For this review, take the finished solid that the model builds, in its own axes (mm). A direction names the side the tool comes from. Give positions to 0.01 mm unless a question says otherwise; leave off trailing zeros. Order: outer loops, then holes, each group sorted by start corner. A loop starts at its lowest first (then second) coordinate and runs counter-clockwise, first axis right, second up. Notation, with made-up numbers: (56.5, 57) - (109.5, 57) arc R22 cw to (109.5, 84) - close; hole circle Ø9 at (53, -22). An arc over 180 degrees is marked (long way). One line per item, written item: value.
```python
from build123d import *

# Parameters (mm, degrees)
BOSS_EXTRUDE1_DEPTH = 2.5
SKETCH2_R           = 5.25
CUT_EXTRUDE1_DEPTH  = 86.727569626


with BuildPart() as part:
    # Sketch1 → Boss-Extrude1 (new, symmetric)
    with BuildSketch(Plane.XY):
        with BuildLine():
            Line((-49.57019439, -4), (-20, -4))
            ThreePointArc((-20, -4), (-17.171572875, -5.171572875), (-16, -8))
            Line((-16, -8), (-16, -19.403091525))
            Line((-16, -19.403091525), (-13.500700251, -20.50145429))
            Line((-13.500700251, -20.50145429), (-16, -24.97))
            Line((-16, -24.97), (-16, -66))
            Line((-16, -66), (0, -66))
            Line((0, -66), (0, 66))
            Line((0, 66), (-15, 66))
            Line((-15, 66), (-15, 62.56))
            ThreePointArc((-15, 62.56), (-26.17355239, 31.809747222), (-54.481338034, 15.405613876))
            ThreePointArc((-54.481338034, 15.405613876), (-50.022346721, 6.209829337), (-49.57019439, -4))
        make_face()
    extrude(amount=BOSS_EXTRUDE1_DEPTH, both=True)

    # Sketch2 → Cut-Extrude1 (cut, through all)
    with BuildSketch(Plane.XY.offset(2.5)):
        with Locations((-8, 51)):
            Circle(SKETCH2_R)
        with Locations((-8, -54)):
            Circle(SKETCH2_R)
    extrude(amount=-CUT_EXTRUDE1_DEPTH, mode=Mode.SUBTRACT)


solid = part.part
```
(1) Take a section at A-A (y = -54). Write out the cut boundary in (x, z).
Answers below:
outline: (-16, -2.5) - (-13.25, -2.5) - (-13.25, 2.5) - (-16, 2.5) - close; (-2.75, -2.5) - (0, -2.5) - (0, 2.5) - (-2.75, 2.5) - close
(2) Wall thickness on line 1 (Y direction, x = -8, z = -0.8); line 2 (Y direction, x = -9.5, z = 0.3); line 3 (X direction, y = -19, z = 0.7): over which ranges is each line inside the solid? List them lowest first. Write a range as from..to.
Answers below:
line 1: y = -66..-59.25, -48.75..45.75, 56.25..66
line 2: y = -66..-59.03, -48.97..45.97, 56.03..66
line 3: x = -16..0
(3) For P1, Ø17, axis at x = -8, y = -54, coming from the +Z side; P2, Ø6.5, axis at x = -8, y = 51, coming from the +Z side; P3, Ø1.5, axis at y = -36, z = 0, coming from the -X side; P4, Ø1.5, axis at x = -38, z = 0.5, coming from the +Y side, all flat-tipped, find the tip position at first contact; note any pin that passes through.
Answers below:
P1: stops at z = 2.5
P2: passes through
P3: stops at x = -16
P4: stops at y = 22.11
(4) Take a section at D-D (y = -14). Write out the cut boundary in (x, z), then the cut area to 3 significant figures.
Answers below:
outline: (-16, -2.5) - (0, -2.5) - (0, 2.5) - (-16, 2.5) - close
area: 80.0 mm^2
(5) Take a section at C-C (z = -0.25). Write out the cut boundary in (x, y).
Answers below:
outline: (-54.48, 15.41) arc R25.27 cw to (-49.57, -4) - (-20, -4) arc R4 cw to (-16, -8) - (-16, -19.4) - (-13.5, -20.5) - (-16, -24.97) - (-16, -66) - (0, -66) - (0, 66) - (-15, 66) - (-15, 62.56) arc R47.9 cw to start; hole circle Ø10.5 at (-8, -54); hole circle Ø10.5 at (-8, 51)
(6) Machinability: for faces 1 (the face through (-15, 64, 0)), 2 (the face through (-14.768, -19.945, 0.035)), 3 (the face through (-16, 1, 2.5)), 4 (the face through (-35, -4, 0)), 5 (the face through (-5.58, -58.66, 0.04)), which of the approach directions +Z, -Z, +X, -X, +Y, -Y give a long, thin tool a straight path to every point of the face, cutting with its end or side? Answer none if there is none.
Answers below:
face 1: +Z, -Z, -X, +Y
face 2: +Z, -Z, -X
face 3: +Z, +X, -X, +Y, -Y
face 4: +Z, -Z, -X, -Y
face 5: +Z, -Z
(7) Draft analysis for pull direction X (two halves, no side actions). For faces 6 (the face through (-5.18, 55.43, 0.04)), 7 (the face through (-16, -45, 0)), 8 (the face through (0, -1, 0)), state which applies: pulls with the +X half, pulls with the -X half, needs draft (parallel to the pull), parting line crosses it, or undercut.
Answers below:
face 6: undercut
face 7: pulls with the -X half
face 8: pulls with the +X half
(8) Take a section at B-B (x = -8). Write out the cut boundary in (y, z).
Answers below:
outline: (-66, -2.5) - (-59.25, -2.5) - (-59.25, 2.5) - (-66, 2.5) - close; (-48.75, -2.5) - (45.75, -2.5) - (45.75, 2.5) - (-48.75, 2.5) - close; (56.25, -2.5) - (66, -2.5) - (66, 2.5) - (56.25, 2.5) - close
